Read the model definition and answer for the solid it produces. Units are mm, in the model's axes. A direction names the side the tool comes from. Give positions to 0.01 mm unless a question says otherwise; leave off trailing zeros. Order: outer loops, then holes, each group sorted by start corner. A loop starts at its lowest first (then second) coordinate and runs counter-clockwise, first axis right, second up.
```python
from build123d import *

# Parameters (mm, degrees)
F1_DEPTH = 100
F2_T     = -2.5
F3_R     = 5


with BuildPart() as f1:
    # F0 (on Front) → F1 (new body)
    with BuildSketch(Plane.XZ):
        Polygon((47.3136231303, -35.2433100343), (49.9879084527, 55.1212131977), (-48.6377365887, 55.1212131977), (-48.6377365887, -35.2433100343), align=None)
    extrude(amount=F1_DEPTH)

    # F2
    f2_openings = [f1.faces().sort_by_distance(p)[0] for p in [
        (0.009578, -100, 10.145948),
    ]]
    offset(amount=F2_T, openings=f2_openings)

    # F3
    f3_edges = [f1.edges().sort_by_distance(p)[0] for p in [
        (-48.637737, -50, 55.121213),
        (47.412828, -51.25, 52.621213),
        (-48.637737, -50, -35.24331),
        (47.313623, -50, -35.24331),
    ]]
    fillet(f3_edges, radius=F3_R)


solid = f1.part
```
1) Consider L1, parallel to Z at x = -30, y = -25; L2, parallel to Y at x = -30, z = -11; L3, parallel to X at y = -90, z = 9.5. Determine where each line is inside the solid, lowest interval first.
Final values:
L1: z = -35.24 to -32.74, 52.62 to 55.12
L2: y = -2.5 to 0
L3: x = -48.64 to -46.14, 46.14 to 48.64
2) The part is cut by section B-B on x = -36.5. Determine the outline of the cut face in (y, z), and give its area (3 significant figures).
Final values:
outline: (-100, -35.24) - (0, -35.24) - (0, 55.12) - (-100, 55.12) - (-100, 52.62) - (-2.5, 52.62) - (-2.5, -32.74) - (-100, -32.74) - close
area: 713 mm2
3) The part is cut by section C-C on z = 40. Determine the outline of the cut face in (x, y), and give its area (3 significant figures).
Final values:
outline: (-48.64, -100) - (-46.14, -100) - (-46.14, -2.5) - (47.04, -2.5) - (47.04, -100) - (49.54, -100) - (49.54, 0) - (-48.64, 0) - close
area: 733 mm2
4) Given pin 1 (5 mm diameter, centred on x = -11.5, z = -4, fed in from -Y); pin 2 (1.5 mm diameter, centred on y = -83.5, z = 18.5, fed in from +X); pin 3 (2 mm diameter, centred on y = -87, z = 46, fed in from +X), each flat-ended and moving along its own axis, determine where each tip first touches the part or whether it passes through.
Final values:
pin 1: stops at y = -2.5
pin 2: stops at x = 48.93
pin 3: stops at x = 49.75
5) A tool of negligible diameter and unlimited length cuts with its end or side. For faces 4 (the face through (-1, -51, -32.743)), 5 (the face through (-48.638, -49, 11)), from which of +Z, -Z, +X, -X, +Y, -Y can it reach the whole face along a straight path? Write none if from no direction.
Final values:
face 4: -Y
face 5: +Z, -Z, -X, +Y, -Y
6) For a pull along X with two mould halves and no side action, classify faces 1 (the face through (45.89, -51.93, 51.06)), 2 (the face through (-47.13, -50.7, 53.7)), 3 (the face through (4, -49, 55.121)) as released by +X, released by -X, zero draft, split by the parting line, or undercut.
Final values:
face 1: undercut
face 2: released by -X
face 3: zero draft
7) The part is cut by section A-A on y = -11. Determine the outline of the cut face in (x, z), and give its area (3 significant figures).
Final values:
outline: (-48.64, -30.24) arc R5 ccw to (-43.64, -35.24) - (42.46, -35.24) arc R5 ccw to (47.46, -30.39) - (49.99, 55.12) - (-43.64, 55.12) arc R5 ccw to (-48.64, 50.12) - close; hole (-46.14, -32.74) - (44.89, -32.74) - (47.26, 47.47) arc R5 ccw to (42.26, 52.62) - (-46.14, 52.62) - close
area: 903 mm2
